Geometry check sheet. Reference: the model listing, model coordinates, mm. A direction names the side the tool comes from. Give positions to 0.01 mm unless a question says otherwise; leave off trailing zeros. Loops run counter-clockwise (first coordinate to the right, second up) from the corner with the lowest first, then second, coordinate; pieces in that order, holes last. Notation, with made-up numbers: (-33, -24) -> (-2, -24) arc R17 cw to (-2, -4) -> close; hole circle Ø11 at (51, 12). An arc over 180 degrees is marked (long way). Write each question's results on one line, items separated by ' | '. Start each with the question number.
1) Sectioned sample at B-B on x = 18.5. Record the cut outline in (y, z) (1 decimal).
2) Set-up check for faces 4 (the face through (15.507, 2, 21)), 5 (the face through (8, 0.312, 11)), 6 (the face through (-1.152, 1.536, 18.056)), 7 (the face through (8, 6.916, 16)), 8 (the face through (16.42, 1.54, 18.11)): record each of +Z, -Z, +X, -X, +Y, -Y from which the full face is reachable in a straight line by a thin tool's end or side.
3) Scan lines: line 1 (Y direction, x = 8, z = 9.5); line 2 (Y direction, x = 16, z = 14.5); line 3 (Z direction, x = 12.5, y = 2.25). Record each from-to range of solid material in increasing order. Write a range as from..to.
4) Draft check along Z on faces 1 (the face through (-0.241, 2, 21)), 2 (the face through (7, 5, 7.62)), 3 (the face through (-0.241, 2, 14)). Enter one of: pulls with the +Z half, pulls with the -Z half, needs draft (parallel to the pull), parting line crosses it, or undercut.
5) Depth check by flat-ended pin: pin 1 (13.5 mm diameter, centred on x = 13.5, z = 16, fed in from -Y); pin 2 (1.9 mm diameter, centred on y = 2, z = 18, fed in from -X); pin 3 (1.9 mm diameter, centred on x = 1, y = 2, fed in from +Z). Enter the tip coordinate at first touch or a pass-through.
6) Sectioned sample at A-A on z = 9.75. Record the cut outline in (x, y), then the cut area to 3 significant figures.
7) Sectioned sample at C-C on z = 21. Record the cut outline in (x, y), then the cut area to 3 significant figures.
8) Sectioned sample at D-D on y = 5.25. Record the cut outline in (x, z), then the cut area to 3 significant figures.
Autodesk Inventor part; units mm, degrees
ref_plane "YZ Plane" through (0, 0, 0) normal (1, 0, 0) x (0, 1, 0)
ref_plane "XZ Plane" through (0, 0, 0) normal (0, 1, 0) x (-1, 0, 0)
ref_plane "XY Plane" through (0, 0, 0) normal (0, 0, 1) x (1, 0, 0)
sketch "Sketch1" plane through (0, 0, 0) normal (0, 0, 1) x (1, 0, 0)
  line L0 (-6.3366, 6.9163) -> (21.6034, 6.9163)
  line L1 (21.6034, 6.9163) -> (21.6034, -8.3237)
  line L2 (21.6034, -8.3237) -> (-6.3366, -8.3237)
  line L3 (-6.3366, -8.3237) -> (-6.3366, 6.9163)
  point P0 (0, 0)
  dimension "d0" = 27.94
  dimension "d1" = 15.24
extrude "Extrusion1" add sketch "Sketch1" along normal blind 7.62
sketch "Sketch2" plane through (0, 0, 7.62) normal (0, 0, 1) x (1, 0, 0)
  line L0 (-6.3366, 6.9163) -> (-6.3366, -8.3237)
  line L1 (21.6034, -8.3237) -> (21.6034, 6.9163)
  line L2 (21.6034, 0.3123) -> (21.6034, 2.7253)
  line L3 (-6.3366, 2.7253) -> (-6.3366, 0.3123)
  line L4 (21.6034, 6.9163) -> (-6.3366, 6.9163)
  line L5 (-6.3366, -8.3237) -> (21.6034, -8.3237)
  line L6 (0.9631, 2.7253) -> (-0.2406, 2.7253)
  line L7 (-0.2406, 0.3123) -> (0.9631, 0.3123)
  line L8 (-0.2406, 0.3123) -> (-0.2406, 2.7253)
  line L9 (-0.2406, 0.3123) -> (3.0821, 0.3123)
  line L10 (3.0821, 0.3123) -> (3.0821, 2.7253)
  line L11 (3.0821, 2.7253) -> (-0.2406, 2.7253)
  line L12 (-0.2406, 2.7253) -> (-0.2406, 0.3123)
  line L13 (14.3038, 2.7253) -> (15.5074, 2.7253)
  line L14 (15.5074, 0.3123) -> (14.3038, 0.3123)
  line L15 (15.5074, 0.3123) -> (15.5074, 2.7253)
  line L16 (15.5074, 0.3123) -> (12.1847, 0.3123)
  line L17 (12.1847, 0.3123) -> (12.1847, 2.7253)
  line L18 (12.1847, 2.7253) -> (15.5074, 2.7253)
  line L19 (15.5074, 2.7253) -> (15.5074, 0.3123)
  line L20 (-6.3366, -0.7037) -> (21.6034, -0.7037)
  line L21 (-6.3366, 2.7253) -> (21.6034, 2.7253)
  line L22 (21.6034, 2.7253) -> (21.6034, 0.3123)
  line L23 (21.6034, 0.3123) -> (-6.3366, 0.3123)
  line L24 (-6.3366, 0.3123) -> (-6.3366, 2.7253)
  point P0 (0, 0)
  point P1 (-0.2406, 1.5188)
  point P2 (15.2669, 0)
  point P3 (15.5074, 1.5188)
  dimension "d6" = 6.096
extrude "Extrusion2" add sketch "Sketch2" along normal blind 8.7376 contours L6 L11 L10 L9 L7 L8 | L15 L14 L16 L17 L18 L13
sketch "Sketch3" plane through (-0.2406, 2.7253, 7.62) normal (0, 1, 0) x (1, 0, 0)
  line L0 (3.3227, -8.7376) -> (0, -8.7376)
  line L1 (3.3227, -8.7376) -> (0, -8.7376)
  line L2 (-6.096, 7.62) -> (21.844, 7.62)
  line L3 (3.3227, -11.3552) -> (3.3227, -8.7376)
  line L4 (12.4253, -8.7376) -> (15.748, -8.7376)
  line L5 (12.4253, -8.7376) -> (15.748, -8.7376)
  line L6 (12.4253, -11.3552) -> (12.4253, -8.7376)
  line L7 (15.748, 0) -> (15.748, -8.7376)
  arc A0 (15.748, -12.1912) -> (15.748, -8.7376) centre (14.5683, -10.4644) ccw
  line L8 (15.748, -12.1912) -> (12.4253, -12.1912)
  line L9 (12.4253, -12.1912) -> (12.4253, -8.7376)
  line L10 (3.3227, -8.7376) -> (0, -8.7376)
  line L11 (3.3227, -8.7376) -> (0, -8.7376)
  line L12 (3.3227, -11.3552) -> (3.3227, -8.7376)
  arc A1 (0, -8.7376) -> (0, -12.1912) centre (1.1797, -10.4644) ccw
  line L13 (0, -12.1912) -> (3.3227, -12.1912)
  line L14 (3.3227, -12.1912) -> (3.3227, -8.7376)
  point P0 (0.2406, 7.62)
  point P1 (3.0718, -11.3552)
extrude "Extrusion4" add sketch "Sketch2" along normal blind 14.2875 contours L6 L11 L10 L9 L7 L8 | L15 L14 L16 L17 L18 L13
sketch "Sketch4" plane through (-6.3366, 6.9163, 0) normal (0, 1, 0) x (1, 0, 0)
  point P0 (6.3366, 0)
sketch "Sketch5" plane through (0, 0, 7.62) normal (0, 0, 1) x (1, 0, 0)
  line L0 (21.6034, 6.9163) -> (-6.3366, 6.9163)
  line L1 (-6.3366, 15.6735) -> (21.6034, 15.6735)
  line L2 (21.6034, 15.6735) -> (21.6034, 6.9163)
  line L3 (21.6034, 6.9163) -> (-6.3366, 6.9163)
  line L4 (-6.3366, 6.9163) -> (-6.3366, 15.6735)
  point P0 (0, 0)
extrude "Extrusion5" add sketch "Sketch5" along normal blind 17.145 and the other way blind 7.62
extrude "Extrusion6" cut sketch "Sketch2" against normal blind 25.4 contours L20 L1 L5 L0
extrude "Extrusion7" add sketch "Sketch2" along normal blind 4.7625 contours L21 L8 L23 L0 | L1 L23 L15 L21 | L21 L17 L23 L10
extrude "Extrusion8" add sketch "Sketch3" against normal up to surface (2.413 mm away)
properties part number "Attachment3"
Result:
1) outline: (-0.7, 0) -> (15.7, 0) -> (15.7, 24.8) -> (6.9, 24.8) -> (6.9, 7.6) -> (2.7, 7.6) -> (2.7, 12.4) -> (0.3, 12.4) -> (0.3, 7.6) -> (-0.7, 7.6) -> close
2) face 4: +Z, +X, -Y | face 5: +Z, +X, -X, -Y | face 6: -X, -Y | face 7: +Z, +X, -X | face 8: +X, -Y
3) line 1: 0.31..2.73, 6.92..15.67 | line 2: 6.92..15.67 | line 3: 0..21.91
4) face 1: needs draft | face 2: pulls with the +Z half | face 3: undercut
5) pin 1: y = 0.31 | pin 2: x = -1.15 | pin 3: z = 21.91
6) outline: (-6.34, 0.31) -> (21.6, 0.31) -> (21.6, 2.73) -> (-6.34, 2.73) -> close; (-6.34, 6.92) -> (21.6, 6.92) -> (21.6, 15.67) -> (-6.34, 15.67) -> close | area: 312 mm^2
7) outline: (-6.34, 6.92) -> (21.6, 6.92) -> (21.6, 15.67) -> (-6.34, 15.67) -> close; (-0.24, 0.31) -> (3.08, 0.31) -> (3.08, 2.73) -> (-0.24, 2.73) -> close; (12.18, 0.31) -> (15.51, 0.31) -> (15.51, 2.73) -> (12.18, 2.73) -> close | area: 261 mm^2
8) outline: (-6.34, 0) -> (21.6, 0) -> (21.6, 7.62) -> (-6.34, 7.62) -> close | area: 213 mm^2
